The drawing under review shows one solid part. Ordinate dimensions are in mm from its lowest x, y, z. Give positions to 0.01 mm unless a question says otherwise; leave off trailing zeros. Write each loop counter-clockwise with the first axis right and the second up, starting at its lowest first coordinate (ties: lowest second). Pieces come first, ordered by that corner, then holes. Notation, with made-up numbers: (23, 58.25) -> (71, 58.25) arc R23 ccw to (71, 74.25) -> close; hole circle Ø1 at (89, 72.5). An arc over 180 degrees is marked (long way). Use CSV: the item, a comma, the result in double quotes.
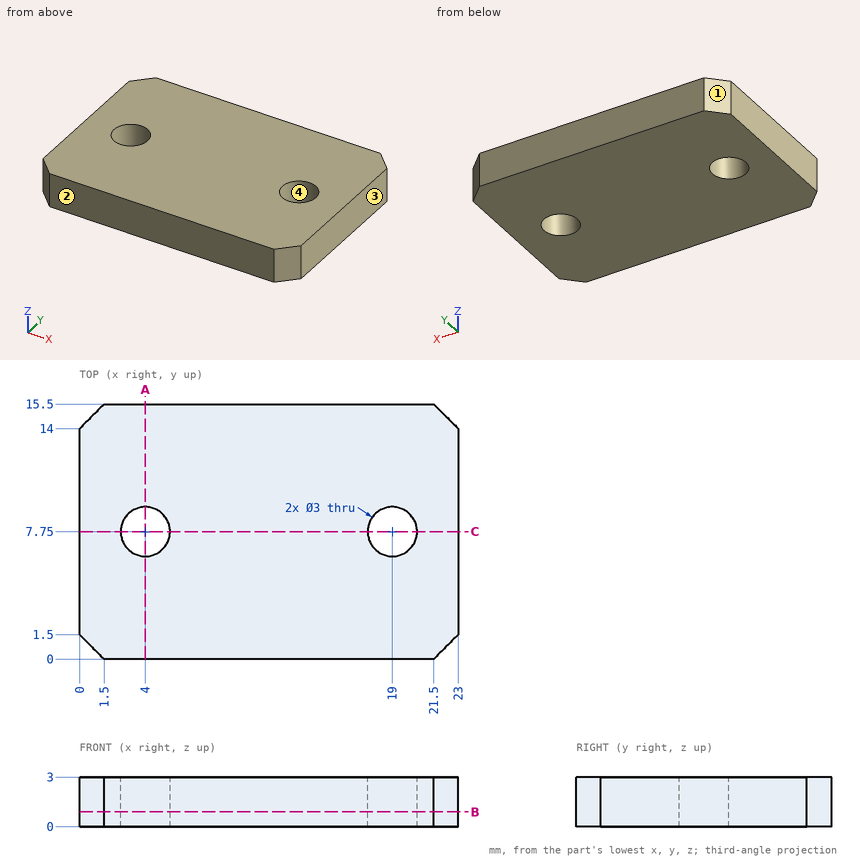
(1) Mouldability with a two-part tool opening along X and no side actions: class the marked faces 1, 2, 3 and 4 as +X half, -X half, draft (parallel to the pull), parting line (faces both ways), or undercut.
Established:
face 1,"-X half"
face 2,"draft"
face 3,"+X half"
face 4,"undercut"
(2) Take a section at B-B (z = 0.9). Write out the cut boundary in (x, y), then the cut area to 3 significant figures.
Established:
outline,"(0, 1.5) -> (1.5, 0) -> (21.5, 0) -> (23, 1.5) -> (23, 14) -> (21.5, 15.5) -> (1.5, 15.5) -> (0, 14) -> close; hole circle Ø3 at (4, 7.75); hole circle Ø3 at (19, 7.75)"
area,"338 mm2"
(3) Clearance check with a flat-ended pin moving along its axis: pin 1 (2.5 mm diameter, centred on x = 19, y = 7.75, fed in from -Z). State where the tip first meets the part, or that it passes through.
Established:
pin 1,"passes through"
(4) Take a section at A-A (x = 4). Write out the cut boundary in (y, z), then the cut area to 3 significant figures.
Established:
outline,"(0, 0) -> (6.25, 0) -> (6.25, 3) -> (0, 3) -> close; (9.25, 0) -> (15.5, 0) -> (15.5, 3) -> (9.25, 3) -> close"
area,"37.5 mm2"
(5) Take a section at C-C (y = 7.75). Write out the cut boundary in (x, z), then the cut area to 3 significant figures.
Established:
outline,"(0, 0) -> (2.5, 0) -> (2.5, 3) -> (0, 3) -> close; (5.5, 0) -> (17.5, 0) -> (17.5, 3) -> (5.5, 3) -> close; (20.5, 0) -> (23, 0) -> (23, 3) -> (20.5, 3) -> close"
area,"51.0 mm2"
(6) For line 1 along X through (y, z) = (7.75, 2.4); line 2 along Y through (x, z) = (19, 1.35); line 3 along X through (y, z) = (6.5, 1.1), list the stretches that pass through material, from the lowest coordinate up. Write a range as [from, to].
Established:
line 1,"x = [0, 2.5], [5.5, 17.5], [20.5, 23]"
line 2,"y = [0, 6.25], [9.25, 15.5]"
line 3,"x = [0, 3.17], [4.83, 18.17], [19.83, 23]"
